For this review, use the dimensioned drawing (mm, ordinates from the lowest corner) and the shaded views. Give positions to 0.01 mm unless a question says otherwise; leave off trailing zeros. Loops run counter-clockwise (first coordinate to the right, second up) from the corner with the lowest first, then second, coordinate; pieces in that order, holes last. Notation, with made-up numbers: (-28, 55.25) -> (6, 55.25) arc R36 cw to (6, 92.25) -> close; hole circle Ø7 at (68, 39). An arc over 180 degrees is marked (long way). Write each question's results on one line, items separated by ' | '. Start each with the question number.
Q1. We need section A-A (z = 2). Write out the cut boundary in (x, y).
Q2. Wall thickness on L1, parallel to Y at x = 5.08, z = 2.5; L2, parallel to Y at x = 5.08, z = 1.05; L3, parallel to X at y = 6.25, z = 4.5 (1 decimal): over which ranges is each line inside the solid? List them lowest first. Write a range as [from, to].
Q3. Mouldability with a two-part tool opening along X and no side actions: class the marked faces 1, 2 and 3 as released by +X, released by -X, zero draft, split by the parting line, or undercut.
Q4. Insertion check: pin 1 Ø3.5 at (x, y) = (5.08, 5.08) entering from +Z; pin 2 Ø1 at (y, z) = (3.5, 5) entering from -X; pin 3 Ø1.5 at (x, z) = (2.5, 2) entering from -Y. Each pin has a flat end and moves straight along its axis. Give the tip position at first contact, or say it passes through.
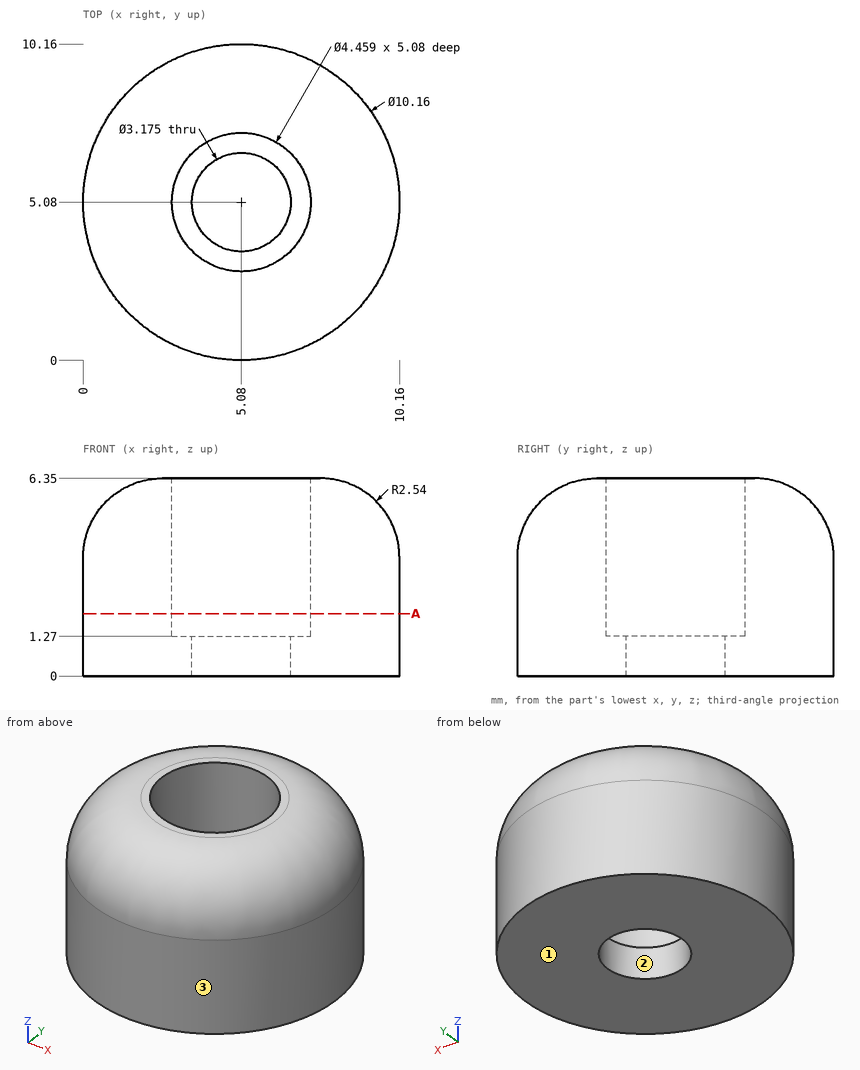
Output:
1) outline: circle Ø10.16 at (5.08, 5.08); hole circle Ø4.46 at (5.08, 5.08)
2) L1: [0, 2.85], [7.31, 10.16] | L2: [0, 3.49], [6.67, 10.16] | L3: [0.2, 3.2], [7, 9.9]
3) face 1: zero draft | face 2: undercut | face 3: split by the parting line
4) pin 1: z = 1.27 | pin 2: x = 0.29 | pin 3: y = 0.34
